Design review of the part built by this model. Coordinates are the model's own, in mm. A direction names the side the tool comes from. Coordinates: 2 decimals unless noted, no trailing zeros. Order: outer loops, then holes, each group sorted by start corner. A loop starts at its lowest first (then second) coordinate and runs counter-clockwise, first axis right, second up. Notation, with made-up numbers: M 31,29.5 L 52,29.5 A26 ccw 52,53.5 Z; hole C 31.25,75 d9. An arc over 180 degrees is marked long. Answer as a JSON object with one key per item and string values.
from build123d import *

# Parameters (mm, degrees)
SKETCH1_W           = 42
SKETCH1_H           = 54
BOSS_EXTRUDE1_DEPTH = 12
CHAMFER2_SIZE       = 12
BOSS_EXTRUDE2_DEPTH = 12
BOSS_EXTRUDE3_DEPTH = 6


with BuildPart() as part:
    # Sketch1 → Boss-Extrude1 (new body)
    with BuildSketch(Plane(origin=(0, 0, 0), x_dir=(1, 0, 0), z_dir=(0, 1, 0))):
        Rectangle(SKETCH1_W, SKETCH1_H)
    extrude(amount=BOSS_EXTRUDE1_DEPTH)

    # Chamfer2
    chamfer2_edges = [part.edges().sort_by_distance(p)[0] for p in [
        (21, 6, 27),
        (-21, 6, 27),
    ]]
    chamfer(chamfer2_edges, length=CHAMFER2_SIZE)

    # Sketch2 → Boss-Extrude2 (add)
    with BuildSketch(Plane(origin=(0, 0, -27), x_dir=(-1, 0, 0), z_dir=(0, 0, -1))):
        with BuildLine():
            Line((21, 0), (21, -27))
            ThreePointArc((21, -27), (0, -48), (-21, -27))
            Line((-21, -27), (-21, 0))
            Line((-21, 0), (21, 0))
        make_face()
    extrude(amount=-BOSS_EXTRUDE2_DEPTH)

    # Sketch8 → Boss-Extrude3 (add, symmetric)
    with BuildSketch(Plane(origin=(0, 0, 0), x_dir=(0, 0, -1), z_dir=(1, 0, 0))):
        Polygon((15, -42), (15, 0), (-27, 0), align=None)
    extrude(amount=BOSS_EXTRUDE3_DEPTH, both=True)


solid = part.part
1) Tool access review of faces 1 (the flat face through (-14, 0, 6)), 2 (the flat face through (6, -11, -3)), 3 (the flat face through (-15, 6, 21)), 4 (the flat face through (0, 6, 27)), 5 (the flat face through (-10, -24, -15)): name each direction out of +Z, -Z, +X, -X, +Y, -Y from which nothing blocks a thin tool from reaching the whole face with its end or side.
Taken from the geometry:
{"face 1": "+Z, -X, -Y", "face 2": "+Z, +X, -Y", "face 3": "+Z, -X, +Y, -Y", "face 4": "+Z, +X, -X, +Y, -Y", "face 5": "+Z, -Y"}
2) Add section B-B (x = 0). State the section outline as (y, z) points.
Taken from the geometry:
{"outline": "M -48,-27 L 12,-27 L 12,27 L 0,27 L -42,-15 L -48,-15 Z"}
3) Add section A-A (z = 22.5). State the section outline as (x, y) points.
Taken from the geometry:
{"outline": "M -13.5,0 L -6,0 L -6,-4.5 L 6,-4.5 L 6,0 L 13.5,0 L 13.5,12 L -13.5,12 Z"}
4) Add section C-C (y = -34). State the section outline as (x, z) points, and give its area (3 significant figures).
Taken from the geometry:
{"outline": "M -19.8,-27 L 19.8,-27 L 19.8,-15 L 6,-15 L 6,-7 L -6,-7 L -6,-15 L -19.8,-15 Z", "area": "571 mm2"}
5) Insertion check: pin 1 Ø1.5 at (x, z) = (2, 12.5) entering from -Y; pin 2 Ø4 at (x, y) = (5, -39) entering from +Z; pin 3 Ø12.5 at (y, z) = (-11, -0.5) entering from -X. Each pin has a flat end and moves straight along its axis. Give the tip position at first contact, or say it passes through.
Taken from the geometry:
{"pin 1": "stops at y = -15.25", "pin 2": "stops at z = -10", "pin 3": "stops at x = -6"}
6) To check wall thickness, follow L1, parallel to Z at x = 11, y = -24; L2, parallel to Y at x = -19, z = 15.5; L3, parallel to X at y = -2, z = -9. State the ranges of each line that lie inside material, in increasing order.
Taken from the geometry:
{"L1": "z = -27 to -15", "L2": "y = 0 to 12", "L3": "x = -6 to 6"}
7) Add section D-D (x = -14). State the section outline as (y, z) points.
Taken from the geometry:
{"outline": "M -42.65,-27 L 12,-27 L 12,22 L 0,22 L 0,-15 L -42.65,-15 Z"}
